```python
from build123d import *

# Parameters (mm, degrees)
F0_R          = 9.525
F0_R_2        = 6.985
F1_DEPTH      = 76.2
F2_R          = 8.690434
F3_DEPTH      = 50.8
F5_DEPTH      = 1.27
F5_DEPTH_BACK = 1.27
F6_R          = 6.985
F7_DEPTH      = 76.2
F8_W          = 76.2
F8_H          = 19.05
F10_R         = 4.445
F11_DEPTH     = 50.8
F12_DEPTH     = 87.884
F13_R         = 1.905
F14_DEPTH     = 12.7


with BuildPart() as f1:
    # F0 (on Top) → F1 (new body)
    with BuildSketch(Plane.XY):
        Circle(F0_R)
        Circle(F0_R_2, mode=Mode.SUBTRACT)
    extrude(amount=F1_DEPTH)

    # F2 (on Front) → F3 (join)
    with BuildSketch(Plane.XZ):
        with Locations((0, 38.1)):
            Circle(F2_R)
    extrude(amount=F3_DEPTH)

    # F4 (on Right) → F5 (join, two sides)
    with BuildSketch(Plane.YZ) as f5_sk:
        Polygon((-50.8, 72.39), (-50.8, 46.99), (-25.4, 46.99), (-25.4, 54.61), align=None)
        Polygon((-25.4, 46.99), (-50.8, 46.99), (-50.647298, 8.890306), (-25.4, 19.05), align=None)
    extrude(amount=F5_DEPTH)
    extrude(f5_sk.sketch, amount=-F5_DEPTH_BACK)

    # F6 (on Top) → F7 (cut)
    with BuildSketch(Plane.XY):
        Circle(F6_R)
    extrude(amount=F7_DEPTH, mode=Mode.SUBTRACT)

    # F8 (on Right) → F9 (revolve)
    with BuildSketch(Plane.YZ):
        with Locations((38.1, 45.344532)):
            Rectangle(F8_W, F8_H)
    revolve(axis=Axis((0, 44.6622, 35.819532), (0, 1, 0)))

    # F10 (on face) → F11 (cut)
    with BuildSketch(Plane(origin=(0, 76.2, 0), x_dir=(-1, 0, 0), z_dir=(0, 1, 0))):
        with Locations((0, 35.819532)):
            Circle(F10_R)
    extrude(amount=-F11_DEPTH, mode=Mode.SUBTRACT)

    # F6 (on Top) → F12 (cut)
    with BuildSketch(Plane.XY):
        Circle(F6_R)
    extrude(amount=F12_DEPTH, mode=Mode.SUBTRACT)

    # F13 (on Front) → F14 (cut)
    with BuildSketch(Plane.XZ):
        with Locations((0, 38.175505)):
            Circle(F13_R)
    extrude(amount=-F14_DEPTH, mode=Mode.SUBTRACT)


solid = f1.part
```
The listing builds one solid part. Answer for the finished solid, in the listing's coordinates (mm). A direction names the side the tool comes from. Give positions to 0.01 mm unless a question says otherwise; leave off trailing zeros. Loops run counter-clockwise (first coordinate to the right, second up) from the corner with the lowest first, then second, coordinate; pieces in that order, holes last. Notation, with made-up numbers: (22.5, 14.25) - (79.5, 14.25) arc R9 ccw to (79.5, 26.25) - close; hole circle Ø9 at (29.5, 5). An arc over 180 degrees is marked (long way). Return JSON: item names as keys, results as strings. Group by question number.
1. Find section A-A (z = 22.5). Write down the section's boundary in (x, y) (3 decimals).
2. Determine the mould class of faces 4 (the flat face through (-0.8, 7.1, 76.2)), 5 (the flat face through (0, -50.8, 60)), 6 (the cylindrical face through (0.96, 51.16, 31.48)), 7 (the flat face through (-0.8, 7.1, 0)) for opening direction Z: pulls with the +Z half, pulls with the -Z half, needs draft (parallel to the pull), parting line crosses it, or undercut.
3. Find section D-D (y = -31.5). Write down the section's boundary in (x, z).
4. Straight lines are drawn through the part: line 1 (Y direction, x = 0, z = 50) (3 decimals); line 2 (Z direction, x = 0, y = 58); line 3 (Y direction, x = 0, z = 34) (3 decimals). For each, find the intervals that lie inside material, in ascending order. Write a range as [from, to].
5. Which of the six approach directions +Z, -Z, +X, -X, +Y, -Y give full straight-line access (tool end or side, diameter ignored) to faces 1 (the flat face through (0, 12.7, 38)), 2 (the flat face through (0, 25.4, 36)), 3 (the flat face through (0, -25.4, 24))?
6. Find section C-C (y = -2.5). Write down the section's boundary in (x, z).
7. Given pin 1 Ø8 at (x, y) = (11.5, -16.5) entering from +Z; pin 2 Ø5 at (x, z) = (15, 36.5) entering from -Y; pin 3 Ø5.5 at (x, z) = (0, 35.82) entering from +Y, each flat-ended and moving along its own axis, determine where each tip first touches the part or whether it passes through.
Verdict:
{
 "1": {"outline": "(-13.62, 0) - (-9.525, 0) arc R9.525 ccw to (9.525, 0) - (13.62, 0) - (13.62, 76.2) - (-13.62, 76.2) - close; (-1.27, -50.702) - (1.27, -50.702) - (1.27, -25.4) - (-1.27, -25.4) - close; hole circle Ø13.97 at (0, 0)"},
 "2": {"face 4": "pulls with the +Z half", "face 5": "needs draft", "face 6": "undercut", "face 7": "pulls with the -Z half"},
 "3": {"outline": "(-1.27, 16.6) - (1.27, 16.6) - (1.27, 29.5) arc R8.69 ccw to (1.27, 46.7) - (1.27, 58.88) - (-1.27, 58.88) - (-1.27, 46.7) arc R8.69 ccw to (-1.27, 29.5) - close"},
 "4": {"line 1": "y = [-50.8, -25.4], [-9.525, -6.985], [6.985, 76.2]", "line 2": "z = [16.77, 31.37], [40.26, 54.87]", "line 3": "y = [-50.8, -6.985], [6.985, 25.4]"},
 "5": {"face 1": "none", "face 2": "+Y", "face 3": "-Z, +X, -X"},
 "6": {"outline": "(-9.19, 0) - (-6.52, 0) - (-6.52, 76.2) - (-9.19, 76.2) - close; (6.52, 0) - (9.19, 0) - (9.19, 76.2) - (6.52, 76.2) - close"},
 "7": {"pin 1": "stops at z = 42.49", "pin 2": "stops at y = 0", "pin 3": "stops at y = 25.4"}
}
